Source: CAD feature listing. Evaluate the final solid. Frame: model axes, mm. A direction names the side the tool comes from. Give positions to 0.01 mm unless a question says otherwise; leave off trailing zeros. Write each loop counter-clockwise with the first axis right and the second up, starting at its lowest first coordinate (ties: lowest second). Pieces come first, ordered by that corner, then holes. Notation, with made-up numbers: (-26.5, 84) -> (-13.5, 84) arc R31 ccw to (-13.5, 123) -> close; hole circle Ø6 at (73, 7.5). An arc over 180 degrees is marked (long way). Use one line per item in the form item = value. Start each with the question number.
(1) Draft query along Y for faces 5 (the face through (-67.703, 19.145, 0.105)), 6 (the face through (-42.703, -0.217, -11.645)), 7 (the face through (-67.101, 16.26, -11.074)). Return one class per face: pulls with the +Y half, pulls with the -Y half, needs draft (parallel to the pull), parting line crosses it, or undercut.
(2) Material intervals for line 1 along Y through (x, z) = (-48, -2.5); line 2 along Y through (x, z) = (-5.5, -0.5); line 3 along Z through (x, y) = (-1, -12), sorted ascending. Write a range as from..to.
(3) Cut plane A-A, the plane z = 0. Output: boundary loops of the cut face in (x, y).
(4) Cut plane C-C, the plane y = 0. Count the separate pieces of the cut face and the enclosed holes in it, and give its area (3 significant figures).
(5) First-contact query: P1, Ø12, axis at x = -41.5, y = 6.5, coming from the +Z side; P2, Ø15, axis at y = 5.5, z = -3, coming from the -X side; P3, Ø1, axis at x = -12.5, z = 0, coming from the -Y side; P4, Ø3, axis at y = 9.5, z = -6, coming from the -X side. Flat tips, straight axial feed; report the tip coordinate or a pass-through.
(6) Cut plane B-B, the plane z = -5.5. Output: boundary loops of the cut face in (x, y).
(7) Set-up query: faces 1 (the face through (-51.94, 13.4, -11.64)), 2 (the face through (-59.102, -0.175, 0.132)), 3 (the face through (-67.703, 13.355, -0.105)), 4 (the face through (-52.27, -13.4, 11.64)). Return all of +Z, -Z, +X, -X, +Y, -Y with unobstructed straight access to the full face (end or side cutting, diameter ignored); none if empty.
from build123d import *

# Parameters (mm, degrees)
F0_R         = 3
F1_DEPTH     = 12.5
F2_R         = 3
F3_DEPTH     = 40
F4_R         = 3
F5_T1_DEPTH  = 7.5
F5_T3_DEPTH  = 7.5
F5_T6_ANGLE  = 90
F5_T8_ANGLE  = 90
F5_T10_ANGLE = 90
F5_T12_ANGLE = 90
F5_T14_ANGLE = 90
F5_T16_ANGLE = 90
F5_T18_ANGLE = 90
F5_T20_ANGLE = 90


# Not quite as in the source:
# - a fillet or chamfer that OpenCascade refuses, or shapes differently, is made with other operations: its cross-section is extruded or revolved along the edge and cut away or added


with BuildPart() as f1:
    # F0 (on Top) → F1 (new body, symmetric)
    with BuildSketch(Plane.XY):
        with BuildLine():
            Line((-68.6048818245, -20), (-13.6048818245, -20))
            ThreePointArc((-13.6048818245, -20), (-33.6048818245, 0), (-13.6048818245, 20))
            Line((-13.6048818245, 20), (-68.6048818245, 20))
            Line((-68.6048818245, 20), (-68.6048818245, 12.5))
            Line((-68.6048818245, 12.5), (-43.6048818245, 12.5))
            Line((-43.6048818245, 12.5), (-43.6048818245, -12.5))
            Line((-43.6048818245, -12.5), (-68.6048818245, -12.5))
            Line((-68.6048818245, -12.5), (-68.6048818245, -20))
        make_face()
        with BuildLine():
            ThreePointArc((-13.6048818245, 20), (-33.6048818245, 0), (-13.6048818245, -20))
            ThreePointArc((-13.6048818245, -20), (0.5372537993, -14.1421356237), (6.3951181755, 0))
            ThreePointArc((6.3951181755, 0), (0.5372537993, 14.1421356237), (-13.6048818245, 20))
        make_face()
        with Locations((-13.6048818245, 0)):
            Circle(F0_R, mode=Mode.SUBTRACT)
    extrude(amount=F1_DEPTH, both=True)

    # F2 (on face) → F3 (join, through all)
    with BuildSketch(Plane.XZ.offset(20)):
        with Locations((-56.1048818245, 0)):
            Circle(F2_R)
    extrude(amount=-F3_DEPTH)

    # F4
    f4_edges = [f1.edges().sort_by_distance(p)[0] for p in [
        (-41.104882, 20, 12.5),
        (-43.604882, 0, 12.5),
        (-56.104882, 12.5, 12.5),
        (-56.104882, -12.5, 12.5),
        (6.395118, 0, -12.5),
        (-43.604882, 0, -12.5),
        (-68.604882, -12.5, 0),
        (-68.604882, 12.5, 0),
        (-56.104882, 12.5, -12.5),
        (-56.104882, -12.5, -12.5),
        (-68.604882, -20, 0),
        (-68.604882, 20, 0),
        (-41.104882, -20, -12.5),
        (-41.104882, -20, 12.5),
        (-41.104882, 20, -12.5),
        (6.395118, 0, 12.5),
    ]]
    fillet(f4_edges, radius=F4_R)

    # F5: fillet of radius 5 on 4 edges, made by hand

    # F5_s2 → F5_t1 (cut)
    with BuildSketch(Plane.XZ.offset(-20)):
        with BuildLine():
            ThreePointArc((-63.6048818245, 12.5), (-67.1404157304, 11.0355339059), (-68.6048818245, 7.5))
            Line((-68.6048818245, 7.5), (-68.6048818245, 12.5))
            Line((-68.6048818245, 12.5), (-63.6048818245, 12.5))
        make_face()
        with BuildLine():
            ThreePointArc((-63.6048818245, -12.5), (-67.1404157304, -11.0355339059), (-68.6048818245, -7.5))
            Line((-68.6048818245, -7.5), (-68.6048818245, -12.5))
            Line((-68.6048818245, -12.5), (-63.6048818245, -12.5))
        make_face()
    extrude(amount=F5_T1_DEPTH, mode=Mode.SUBTRACT)

    # F5_s4 → F5_t3 (cut)
    with BuildSketch(Plane.XZ.offset(12.5)):
        with BuildLine():
            ThreePointArc((-63.6048818245, -12.5), (-67.1404157304, -11.0355339059), (-68.6048818245, -7.5))
            Line((-68.6048818245, -7.5), (-68.6048818245, -12.5))
            Line((-68.6048818245, -12.5), (-63.6048818245, -12.5))
        make_face()
        with BuildLine():
            ThreePointArc((-63.6048818245, 12.5), (-67.1404157304, 11.0355339059), (-68.6048818245, 7.5))
            Line((-68.6048818245, 7.5), (-68.6048818245, 12.5))
            Line((-68.6048818245, 12.5), (-63.6048818245, 12.5))
        make_face()
    extrude(amount=F5_T3_DEPTH, mode=Mode.SUBTRACT)

    # F5_s5 → F5_t6 (revolve, cut)
    with BuildSketch(Plane.XY.offset(7.5)):
        with BuildLine():
            ThreePointArc((-65.6048818245, -12.5), (-67.726202168, -13.3786796564), (-68.6048818245, -15.5))
            Line((-68.6048818245, -15.5), (-68.6048818245, -12.5))
            Line((-68.6048818245, -12.5), (-65.6048818245, -12.5))
        make_face()
    revolve(axis=Axis((-63.6048818245, -12.5, 7.5), (0, 1, 0)), revolution_arc=F5_T6_ANGLE, mode=Mode.SUBTRACT)

    # F5_s7 → F5_t8 (revolve, cut)
    with BuildSketch(Plane.YZ.offset(-63.6048818245)):
        with BuildLine():
            ThreePointArc((-20, 9.5), (-19.1213203436, 11.6213203436), (-17, 12.5))
            Line((-17, 12.5), (-20, 12.5))
            Line((-20, 12.5), (-20, 9.5))
        make_face()
    revolve(axis=Axis((-63.6048818245, -20, 7.5), (0, -1, 0)), revolution_arc=F5_T8_ANGLE, mode=Mode.SUBTRACT)

    # F5_s9 → F5_t10 (revolve, cut)
    with BuildSketch(Plane.YZ.offset(-63.6048818245)):
        with BuildLine():
            ThreePointArc((-12.5, -9.5), (-13.3786796564, -11.6213203436), (-15.5, -12.5))
            Line((-15.5, -12.5), (-12.5, -12.5))
            Line((-12.5, -12.5), (-12.5, -9.5))
        make_face()
    revolve(axis=Axis((-63.6048818245, -12.5, -7.5), (0, 1, 0)), revolution_arc=F5_T10_ANGLE, mode=Mode.SUBTRACT)

    # F5_s11 → F5_t12 (revolve, cut)
    with BuildSketch(Plane.XY.offset(-7.5)):
        with BuildLine():
            ThreePointArc((-65.6048818245, -20), (-67.726202168, -19.1213203436), (-68.6048818245, -17))
            Line((-68.6048818245, -17), (-68.6048818245, -20))
            Line((-68.6048818245, -20), (-65.6048818245, -20))
        make_face()
    revolve(axis=Axis((-63.6048818245, -20, -7.5), (0, -1, 0)), revolution_arc=F5_T12_ANGLE, mode=Mode.SUBTRACT)

    # F5_s13 → F5_t14 (revolve, cut)
    with BuildSketch(Plane.YZ.offset(-63.6048818245)):
        with BuildLine():
            ThreePointArc((20, -9.5), (19.1213203436, -11.6213203436), (17, -12.5))
            Line((17, -12.5), (20, -12.5))
            Line((20, -12.5), (20, -9.5))
        make_face()
    revolve(axis=Axis((-63.6048818245, 20, -7.5), (0, 1, 0)), revolution_arc=F5_T14_ANGLE, mode=Mode.SUBTRACT)

    # F5_s15 → F5_t16 (revolve, cut)
    with BuildSketch(Plane.XY.offset(-7.5)):
        with BuildLine():
            ThreePointArc((-65.6048818245, 12.5), (-67.726202168, 13.3786796564), (-68.6048818245, 15.5))
            Line((-68.6048818245, 15.5), (-68.6048818245, 12.5))
            Line((-68.6048818245, 12.5), (-65.6048818245, 12.5))
        make_face()
    revolve(axis=Axis((-63.6048818245, 12.5, -7.5), (0, -1, 0)), revolution_arc=F5_T16_ANGLE, mode=Mode.SUBTRACT)

    # F5_s17 → F5_t18 (revolve, cut)
    with BuildSketch(Plane.XY.offset(7.5)):
        with BuildLine():
            ThreePointArc((-65.6048818245, 20), (-67.726202168, 19.1213203436), (-68.6048818245, 17))
            Line((-68.6048818245, 17), (-68.6048818245, 20))
            Line((-68.6048818245, 20), (-65.6048818245, 20))
        make_face()
    revolve(axis=Axis((-63.6048818245, 20, 7.5), (0, 1, 0)), revolution_arc=F5_T18_ANGLE, mode=Mode.SUBTRACT)

    # F5_s19 → F5_t20 (revolve, cut)
    with BuildSketch(Plane.YZ.offset(-63.6048818245)):
        with BuildLine():
            ThreePointArc((12.5, 9.5), (13.3786796564, 11.6213203436), (15.5, 12.5))
            Line((15.5, 12.5), (12.5, 12.5))
            Line((12.5, 12.5), (12.5, 9.5))
        make_face()
    revolve(axis=Axis((-63.6048818245, 12.5, 7.5), (0, -1, 0)), revolution_arc=F5_T20_ANGLE, mode=Mode.SUBTRACT)


solid = f1.part
Geometry says:
q1.face_5 = pulls with the +Y half
q1.face_6 = undercut
q1.face_7 = needs draft
q2.line_1 = -20..-12.5, 12.5..20
q2.line_2 = -18.28..18.28
q2.line_3 = -12.47..12.47
q3.outline = (-68.6, -17) arc R3 ccw to (-65.6, -20) -> (-13.6, -20) arc R20 ccw to (-13.6, 20) -> (-65.6, 20) arc R3 ccw to (-68.6, 17) -> (-68.6, 15.5) arc R3 ccw to (-65.6, 12.5) -> (-59.1, 12.5) -> (-59.1, -12.5) -> (-65.6, -12.5) arc R3 ccw to (-68.6, -15.5) -> close; hole (-53.1, -12.5) -> (-43.6, -12.5) -> (-43.6, 12.5) -> (-53.1, 12.5) -> close; hole circle Ø6 at (-13.6, 0)
q4.separate_pieces = 3
q4.enclosed_holes = 0
q4.area = 1,120 mm^2
q5.P1 = 12.5
q5.P2 = -67.26
q5.P3 = -19.99
q5.P4 = -43.6
q6.outline = (-68.6, -17) arc R3 ccw to (-65.6, -20) -> (-13.6, -20) arc R20 ccw to (-13.6, 20) -> (-65.6, 20) arc R3 ccw to (-68.6, 17) -> (-68.6, 15.5) arc R3 ccw to (-65.6, 12.5) -> (-43.6, 12.5) -> (-43.6, -12.5) -> (-65.6, -12.5) arc R3 ccw to (-68.6, -15.5) -> close; hole circle Ø6 at (-13.6, 0)
q7.face_1 = -Z, -X
q7.face_2 = none
q7.face_3 = +Z, -Z, -X
q7.face_4 = +Z, -X
